Could you check a few things on this model? Use its own coordinates, in mm. A direction names the side the tool comes from. Round coordinates to 2 decimals unless told otherwise and drop trailing zeros. Write each loop counter-clockwise with the first axis right and the second up, starting at its lowest first coordinate (ties: lowest second). Pieces come first, ordered by that corner, then holes. Notation, with made-up numbers: (22.25, -16.75) - (52.25, -16.75) arc R18 cw to (52.25, 6.25) - close; hole circle Ø3 at (-27, 27). An arc over 180 degrees is marked (long way). Put each result on its own line as item: value.
from build123d import *

# Parameters (mm, degrees)
SKETCH1_W               = 75
SKETCH1_H               = 70
BOSS_EXTRUDE1_DEPTH     = 4
SKETCH4_W               = 26
SKETCH4_H               = 25
BOSS_EXTRUDE2_DEPTH     = 2
SKETCH3_R               = 4.1
CUT_EXTRUDE1_DEPTH      = 22
SKETCH5_W               = 40
SKETCH5_H               = 45
BOSS_EXTRUDE3_DEPTH     = 4
SKETCH7_R               = 11.3
SKETCH7_R_2             = 1.5
CUT_EXTRUDE2_DEPTH      = 86.248167136
SKETCH8_W               = 4
SKETCH8_H               = 25
BOSS_EXTRUDE4_DEPTH     = 4
FILLET2_R               = 4
SKETCH10_W              = 89
SKETCH10_H              = 3
BOSS_EXTRUDE5_DEPTH     = 6
CHAMFER2_SIZE           = 4
FILLET3_R               = 1
SKETCH11_W              = 40
SKETCH11_H              = 53
CUT_EXTRUDE3_DEPTH      = 86.622718948
SKETCH13_W              = 25
SKETCH13_H              = 70
BOSS_EXTRUDE6_DEPTH     = 8
SKETCH14_W              = 41
SKETCH14_H              = 15
CUT_EXTRUDE4_DEPTH      = 56.427881071
FILLET4_R               = 10
SKETCH15_R              = 1.65
CUT_EXTRUDE5_DEPTH      = 10
CUT_EXTRUDE6_DEPTH      = 58.063561053
CUT_EXTRUDE6_DEPTH_BACK = 58.063561053
SKETCH16_R              = 1.65


with BuildPart() as part:
    # Sketch1 → Boss-Extrude1 (new body)
    with BuildSketch(Plane.XY):
        Rectangle(SKETCH1_W, SKETCH1_H)
    extrude(amount=BOSS_EXTRUDE1_DEPTH)

    # Sketch4 → Boss-Extrude2 (add)
    with BuildSketch(Plane.XY.offset(4)):
        with Locations((-24.5, 20)):
            Rectangle(SKETCH4_W, SKETCH4_H)
        with Locations((-24.5, -20)):
            Rectangle(SKETCH4_W, SKETCH4_H)
    extrude(amount=BOSS_EXTRUDE2_DEPTH)

    # Sketch3 → Cut-Extrude1 (cut)
    with BuildSketch(Plane.ZY.offset(37.5)):
        with Locations((6.1, 20)):
            Circle(SKETCH3_R)
        with Locations((6.1, -20)):
            Circle(SKETCH3_R)
    extrude(amount=-CUT_EXTRUDE1_DEPTH, mode=Mode.SUBTRACT)

    # Sketch5 → Boss-Extrude3 (add)
    with BuildSketch(Plane.XY.offset(4)):
        with Locations((57.5, 0)):
            Rectangle(SKETCH5_W, SKETCH5_H)
    extrude(amount=-BOSS_EXTRUDE3_DEPTH)

    # Sketch7 → Cut-Extrude2 (cut, through all)
    with BuildSketch(Plane(origin=(0, 0, 0), x_dir=(-1, 0, 0), z_dir=(0, 0, -1))):
        with Locations((-54.5, 0)):
            Circle(SKETCH7_R)
        with Locations((-70, 15.5)):
            Circle(SKETCH7_R_2)
        with Locations((-39, 15.5)):
            Circle(SKETCH7_R_2)
        with Locations((-39, -15.5)):
            Circle(SKETCH7_R_2)
        with Locations((-70, -15.5)):
            Circle(SKETCH7_R_2)
    extrude(amount=-CUT_EXTRUDE2_DEPTH, mode=Mode.SUBTRACT)

    # Sketch8 → Boss-Extrude4 (add)
    with BuildSketch(Plane.XY.offset(6)):
        with Locations((-13.5, 20)):
            Rectangle(SKETCH8_W, SKETCH8_H)
        with Locations((-13.5, -20)):
            Rectangle(SKETCH8_W, SKETCH8_H)
    extrude(amount=BOSS_EXTRUDE4_DEPTH)

    # Fillet2
    fillet2_edges = [part.edges().sort_by_distance(p)[0] for p in [
        (-13.5, -32.5, 10),
        (-13.5, -7.5, 10),
        (-13.5, 32.5, 10),
        (-13.5, 7.5, 10),
    ]]
    fillet(fillet2_edges, radius=FILLET2_R)

    # Sketch10 → Boss-Extrude5 (add)
    with BuildSketch(Plane.XY.offset(4)):
        with Locations((33, 21)):
            Rectangle(SKETCH10_W, SKETCH10_H)
        with Locations((33, -21)):
            Rectangle(SKETCH10_W, SKETCH10_H)
    extrude(amount=BOSS_EXTRUDE5_DEPTH)

    # Chamfer2
    chamfer2_edges = [part.edges().sort_by_distance(p)[0] for p in [
        (37.5, 22.5, 2),
        (37.5, -22.5, 2),
        (77.5, 22.5, 5),
        (77.5, -22.5, 5),
    ]]
    chamfer(chamfer2_edges, length=CHAMFER2_SIZE)

    # Fillet3
    fillet3_edges = [part.edges().sort_by_distance(p)[0] for p in [
        (76.5, 19.5, 7),
        (76.5, -19.5, 7),
    ]]
    fillet(fillet3_edges, radius=FILLET3_R)

    # Sketch11 → Cut-Extrude3 (cut, through all)
    with BuildSketch(Plane(origin=(0, 0, 0), x_dir=(-1, 0, 0), z_dir=(0, 0, -1))):
        with Locations((-57.5, 0)):
            Rectangle(SKETCH11_W, SKETCH11_H)
    extrude(amount=-CUT_EXTRUDE3_DEPTH, mode=Mode.SUBTRACT)

    # Sketch13 → Boss-Extrude6 (add)
    with BuildSketch(Plane(origin=(37.5, 0, 0), x_dir=(0, 0, -1), z_dir=(1, 0, 0))):
        with Locations((-12.5, 0)):
            Rectangle(SKETCH13_W, SKETCH13_H)
    extrude(amount=-BOSS_EXTRUDE6_DEPTH)

    # Sketch14 → Cut-Extrude4 (cut, through all)
    with BuildSketch(Plane.XY.offset(4)):
        with Locations((9, 0)):
            Rectangle(SKETCH14_W, SKETCH14_H)
    extrude(amount=-CUT_EXTRUDE4_DEPTH, mode=Mode.SUBTRACT)

    # Fillet4
    fillet4_edges = [part.edges().sort_by_distance(p)[0] for p in [
        (33.5, -35, 25),
        (33.5, 35, 25),
    ]]
    fillet(fillet4_edges, radius=FILLET4_R)

    # Sketch15 → Cut-Extrude5 (cut)
    with BuildSketch(Plane(origin=(37.5, 0, 0), x_dir=(0, 0, -1), z_dir=(1, 0, 0))):
        with Locations(Location((-13.7, 0, 0), (0, 0, 90))):
            Circle(SKETCH15_R)
    extrude(amount=-CUT_EXTRUDE5_DEPTH, mode=Mode.SUBTRACT)

    # Sketch16 → Cut-Extrude6 (cut, two sides: drawn at the far end of the back side and taken through both)
    with BuildSketch(Plane(origin=(0, 0, 0), x_dir=(-1, 0, 0), z_dir=(0, 0, -1)).offset(-CUT_EXTRUDE6_DEPTH_BACK)):
        with Locations((31, 28.238089535)):
            Circle(SKETCH16_R)
        with Locations((31, 11.761910465)):
            Circle(SKETCH16_R)
        with Locations(Location((31, -11.761910465, 0), (0, 0, 180))):
            Circle(SKETCH16_R)
        with Locations(Location((31, -28.238089535, 0), (0, 0, 180))):
            Circle(SKETCH16_R)
        with Locations(Location((-14.38196164, 28.5, 0), (0, 0, 180))):
            Circle(SKETCH16_R)
        with Locations(Location((6.92196164, 28.5, 0), (0, 0, 180))):
            Circle(SKETCH16_R)
        with Locations(Location((-13.99696164, -28.5, 0), (0, 0, 180))):
            Circle(SKETCH16_R)
        with Locations(Location((6.53696164, -28.5, 0), (0, 0, 180))):
            Circle(SKETCH16_R)
    extrude(amount=CUT_EXTRUDE6_DEPTH + CUT_EXTRUDE6_DEPTH_BACK, mode=Mode.SUBTRACT)


solid = part.part
(1) Imagine slicing it at D-D, the plane x = -31. Give the number of separate pieces and of enclosed holes in the cut face, then the cut area to 3 significant figures.
Values found:
separate pieces: 5
enclosed holes: 0
area: 250 mm^2
(2) Imagine slicing it at C-C, the plane x = 32. List the corners of the cut face in (y, z) for me.
Values found:
outline: (-35, 0) - (35, 0) - (35, 15) arc R10 ccw to (25, 25) - (-25, 25) arc R10 ccw to (-35, 15) - close; hole circle Ø3.3 at (0, 13.7)
(3) Please list where these lines run through material, in increasing order: probe 1 along X at (y, z) = (-11.5, 5.5); probe 2 along X at (y, z) = (29.5, 3.5); probe 3 along X at (y, z) = (-16, 15). Write a range as from..to.
Values found:
probe 1: x = -37.5..-32.63, -29.37..-11.5, 29.5..37.5
probe 2: x = -37.5..-32.06, -29.94..-8.23, -5.61..13.07, 15.69..37.5
probe 3: x = 29.5..37.5
(4) I'm going to push flat-ended pins straight in: pin 1 (14 mm diameter, centred on x = 2, y = 26.5, fed in from +Z); pin 2 (6.5 mm diameter, centred on x = 0.5, z = 7.5, fed in from +Y); pin 3 (0.6 mm diameter, centred on x = -21.5, z = 5.5, fed in from -Y). Where does each tip first touch, or does it pass through?
Values found:
pin 1: stops at z = 10
pin 2: stops at y = 22.5
pin 3: stops at y = -32.5
(5) Imagine slicing it at B-B, the plane z = 13.7. List the corners of the cut face in (x, y) for me.
Values found:
outline: (29.5, -35) - (37.5, -35) - (37.5, -1.65) - (29.5, -1.65) - close; (29.5, 1.65) - (37.5, 1.65) - (37.5, 35) - (29.5, 35) - close
(6) For faces 1 (the face through (9, 22.5, 7)), 2 (the face through (9, -13, 4)), 3 (the face through (9, -7.5, 2)), 4 (the face through (-25, 0, 4)), 5 (the face through (-13.472, -31.359, 8.797)), which set-ups out of +Z, -Z, +X, -X, +Y, -Y let a thin tool reach every point of the face, with its end or its side?
Values found:
face 1: +Z, +Y
face 2: +Z
face 3: +Z, -Z
face 4: +Z, -X
face 5: +Z, -X, -Y
(7) Imagine slicing it at A-A, the plane x = -1.5. List the corners of the cut face in (y, z) for me, then the cut area to 3 significant figures.
Values found:
outline: (-35, 0) - (-7.5, 0) - (-7.5, 4) - (-19.5, 4) - (-19.5, 10) - (-22.5, 10) - (-22.5, 4) - (-35, 4) - close; (7.5, 0) - (35, 0) - (35, 4) - (22.5, 4) - (22.5, 10) - (19.5, 10) - (19.5, 4) - (7.5, 4) - close
area: 256 mm^2
(8) If we mould it in two halves opening along Z, with no side actions, what happens to faces 6 (the face through (33.6, -0.4, 12.1)), 7 (the face through (-11.5, 27, 7)), 8 (the face through (-27, -20, 2))? For each: pulls with the +Z half, pulls with the -Z half, needs draft (parallel to the pull), parting line crosses it, or undercut.
Values found:
face 6: undercut
face 7: needs draft
face 8: pulls with the +Z half
